```python
from build123d import *

# Parameters (mm, degrees)
SKETCH1_R           = 1.47
BOSS_EXTRUDE1_DEPTH = 1.5875
SKETCH3_W           = 7.175
SKETCH3_H           = 45
CUT_EXTRUDE1_DEPTH  = 4.175


with BuildPart() as part:
    # Sketch1 → Boss-Extrude1 (new body, symmetric)
    with BuildSketch(Plane.XY):
        Polygon((-12.5, 50), (-35, 50), (-35, 12.5), (-38.175, 12.5), (-38.175, -12.5), (-35, -12.5), (-35, -50), (-12.5, -50), (-12.5, -46.825), (-1.47, -46.825), (-1.47, -43.125), (-3.25, -43.125), (-3.25, -40.525), (-1.47, -40.525), (-1.47, -36.825), (1.47, -36.825), (1.47, -40.525), (3.25, -40.525), (3.25, -43.125), (1.47, -43.125), (1.47, -46.825), (12.5, -46.825), (12.5, -50), (35, -50), (35, -12.5), (38.175, -12.5), (38.175, 12.5), (35, 12.5), (35, 50), (12.5, 50), (12.5, 46.825), (1.47, 46.825), (1.47, 43.125), (3.25, 43.125), (3.25, 40.525), (1.47, 40.525), (1.47, 36.825), (-1.47, 36.825), (-1.47, 40.525), (-3.25, 40.525), (-3.25, 43.125), (-1.47, 43.125), (-1.47, 46.825), (-12.5, 46.825), align=None)
        with Locations((-36.5875, 0)):
            Circle(SKETCH1_R, mode=Mode.SUBTRACT)
        with Locations((36.5875, 0)):
            Circle(SKETCH1_R, mode=Mode.SUBTRACT)
    extrude(amount=BOSS_EXTRUDE1_DEPTH, both=True)

    # Sketch3 → Cut-Extrude1 (cut, through all)
    with BuildSketch(Plane(origin=(0, 0, -1.5875), x_dir=(-1, 0, 0), z_dir=(0, 0, -1))):
        with Locations((-15.3, 0)):
            Rectangle(SKETCH3_W, SKETCH3_H)
    extrude(amount=-CUT_EXTRUDE1_DEPTH, mode=Mode.SUBTRACT)


solid = part.part
```
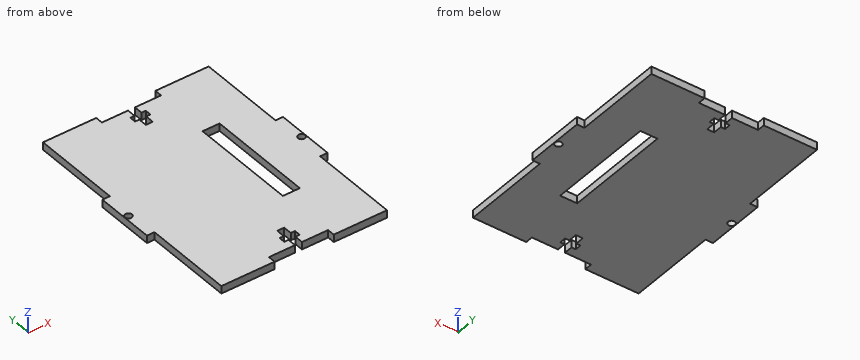
Read the model definition and answer for the solid it produces. Units are mm, in the model's axes. Round coordinates to 2 decimals unless told otherwise and drop trailing zeros. Write each loop counter-clockwise with the first axis right and the second up, starting at its lowest first coordinate (ties: lowest second). Pieces come first, ordered by that corner, then holes. Notation, with made-up numbers: (15, 21.5) - (53, 21.5) arc R26 cw to (53, 40.5) - close; hole circle Ø11 at (-33, 44). An arc over 180 degrees is marked (long way). One line per item, written item: value.
Q1. Find section A-A (y = 9.5). Determine the outline of the cut face in (x, z) (1 decimal), and give its area (3 significant figures).
The answers:
outline: (-38.2, -1.6) - (11.7, -1.6) - (11.7, 1.6) - (-38.2, 1.6) - close; (18.9, -1.6) - (38.2, -1.6) - (38.2, 1.6) - (18.9, 1.6) - close
area: 220 mm2
Q2. Find section B-B (z = -0.2). Count the separate pieces of the cut face and the enclosed holes in it, and give its area (3 significant figures).
The answers:
separate pieces: 1
enclosed holes: 3
area: 6,590 mm2
Q3. Straight lines are drawn through the part: line 1 (X direction, y = 46.5, z = 0.45); line 2 (X direction, y = -1, z = -0.55) (1 decimal); line 3 (X direction, y = -30.5, z = -1.3). For each, find the intervals that lie inside material, in ascending order. Write a range as from..to.
The answers:
line 1: x = -35..-1.47, 1.47..35
line 2: x = -38.2..-37.7, -35.5..11.7, 18.9..35.5, 37.7..38.2
line 3: x = -35..35
Q4. Each of these flat-tipped pins is pushed along its axis until it touches: P1, Ø1.6, axis at y = 48, z = 0.5, coming from the +X side; P2, Ø1.4, axis at x = 2.5, z = 0.5, coming from the -Y side (3 decimals); P3, Ø4, axis at x = 16, y = -18, coming from the +Z side; P4, Ø1.5, axis at x = -11.5, z = 0.5, coming from the +Y side (3 decimals). Where does it stop, or does it pass through?
The answers:
P1: stops at x = 35
P2: stops at y = -46.825
P3: passes through
P4: stops at y = 46.825
